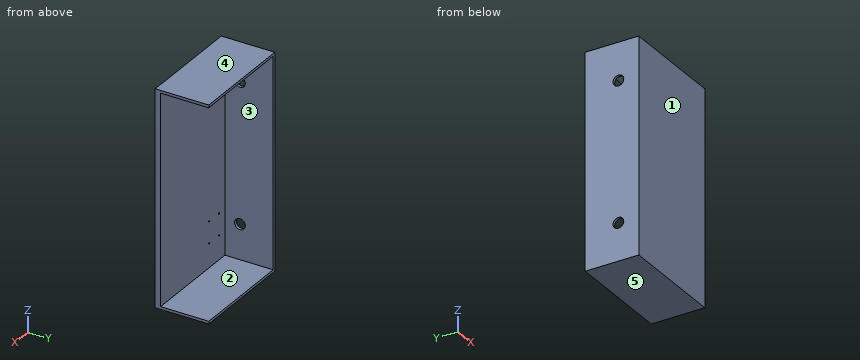
```python
from build123d import *

# Parameters (mm, degrees)
ESQUISSE1_W             = 200
ESQUISSE1_H             = 400
BOSS_EXTRU_1_DEPTH      = 10
BOSS_EXTRU_2_DEPTH      = 90
ENL_V_MAT_EXTRU_1_REACH = 458.098
ESQUISSE3_R             = 10
ESQUISSE4_R             = 1.5
ENL_V_MAT_EXTRU_2_DEPTH = 5


with BuildPart() as part:
    # Esquisse1 → Boss.-Extru.1 (new body)
    with BuildSketch(Plane(origin=(0, 0, 0), x_dir=(1, 0, 0), z_dir=(0, 1, 0))):
        with Locations((100, 200)):
            Rectangle(ESQUISSE1_W, ESQUISSE1_H)
    extrude(amount=BOSS_EXTRU_1_DEPTH)

    # Esquisse2 → Boss.-Extru.2 (add)
    with BuildSketch(Plane(origin=(0, 10, 0), x_dir=(1, 0, 0), z_dir=(0, 1, 0))):
        Polygon((5, 5), (5, 395), (200, 395), (200, 400), (0, 400), (0, 0), (200, 0), (200, 5), align=None)
    extrude(amount=BOSS_EXTRU_2_DEPTH)

    # Esquisse3 → Enlèv. mat.-Extru.1 (cut, up to next)
    with BuildSketch(Plane(origin=(5, 0, 0), x_dir=(0, 0, -1), z_dir=(1, 0, 0)), mode=Mode.PRIVATE) as enl_v_mat_extru_1_sk1:
        with Locations((70, 38)):
            Circle(ESQUISSE3_R)
    enl_v_mat_extru_1_tool1 = extrude(enl_v_mat_extru_1_sk1.sketch, amount=-ENL_V_MAT_EXTRU_1_REACH, mode=Mode.PRIVATE) & part.part
    # Esquisse3 → Enlèv. mat.-Extru.1 (cut, up to next)
    with BuildSketch(Plane(origin=(5, 0, 0), x_dir=(0, 0, -1), z_dir=(1, 0, 0)), mode=Mode.PRIVATE) as enl_v_mat_extru_1_sk2:
        with Locations((330, 38)):
            Circle(ESQUISSE3_R)
    enl_v_mat_extru_1_tool2 = extrude(enl_v_mat_extru_1_sk2.sketch, amount=-ENL_V_MAT_EXTRU_1_REACH, mode=Mode.PRIVATE) & part.part
    add(enl_v_mat_extru_1_tool1.solids().sort_by_distance((5, 38, -70))[0], mode=Mode.SUBTRACT)
    add(enl_v_mat_extru_1_tool2.solids().sort_by_distance((5, 38, -330))[0], mode=Mode.SUBTRACT)

    # Esquisse4 → Enlèv. mat.-Extru.2 (cut)
    with BuildSketch(Plane(origin=(0, 10, 0), x_dir=(1, 0, 0), z_dir=(0, 1, 0))):
        with Locations(Location((23, 350, 0), (0, 0, 270))):
            Circle(ESQUISSE4_R)
        with Locations(Location((53, 350, 0), (0, 0, 270))):
            Circle(ESQUISSE4_R)
        with Locations(Location((53, 310, 0), (0, 0, 270))):
            Circle(ESQUISSE4_R)
        with Locations(Location((23, 310, 0), (0, 0, 270))):
            Circle(ESQUISSE4_R)
        with Locations(Location((23, 90, 0), (0, 0, 90))):
            Circle(ESQUISSE4_R)
        with Locations(Location((53, 90, 0), (0, 0, 90))):
            Circle(ESQUISSE4_R)
        with Locations(Location((53, 50, 0), (0, 0, 90))):
            Circle(ESQUISSE4_R)
        with Locations(Location((23, 50, 0), (0, 0, 90))):
            Circle(ESQUISSE4_R)
    extrude(amount=-ENL_V_MAT_EXTRU_2_DEPTH, mode=Mode.SUBTRACT)


solid = part.part
```
Source: CAD feature listing. Evaluate the final solid. Frame: model axes, mm. Face numbers are marked on the shaded views. A direction names the side the tool comes from. Round coordinates to 2 decimals unless told otherwise and drop trailing zeros. Loops run counter-clockwise (first coordinate to the right, second up) from the corner with the lowest first, then second, coordinate; pieces in that order, holes last.
1. Section query C-C on x = 110.5. Output: boundary loops of the cut face in (y, z).
2. Section query B-B on z = -70. Output: boundary loops of the cut face in (x, y), and give its area (3 significant figures).
3. Mould query, pull axis Z, two halves, no side actions, for the marked faces 3, 4 and 5. Classes: released by +Z, released by -Z, zero draft, split by the parting line, or undercut.
4. Ray query, L1, parallel to X at y = 8.15, z = -350; L2, parallel to Z at x = 154, y = 26.5; L3, parallel to Y at x = 3, z = -330. Return the intervals inside material, ascending.
5. Contact query for flat-ended pins moving along their axis: pin 1 (10 mm diameter, centred on x = 150, z = -115, fed in from +Y); pin 2 (6 mm diameter, centred on y = 34.5, z = -62, fed in from -X); pin 3 (1.8 mm diameter, centred on x = 23, z = -90, fed in from +Y); pin 4 (8 mm diameter, centred on y = 79.5, z = -152.5, fed in from +X). Output: stop coordinate, or through.
6. Section query D-D on y = 76. Output: boundary loops of the cut face in (x, z).
7. Access query for the marked faces 1 and 2. Directions: +Z, -Z, +X, -X, +Y, -Y. A direction counts if a zero-diameter tool reaches every point of the face in a straight line with its end or side. Return the directions, or none.
8. Section query A-A on y = 38. Output: boundary loops of the cut face in (x, z), and give its area (3 significant figures).
Answers below:
1. outline: (0, -400) - (100, -400) - (100, -395) - (10, -395) - (10, -5) - (100, -5) - (100, 0) - (0, 0) - close
2. outline: (0, 0) - (200, 0) - (200, 10) - (5, 10) - (5, 28) - (0, 28) - close; (0, 48) - (5, 48) - (5, 100) - (0, 100) - close
2. area: 2,350 mm2
3. face 3: undercut
3. face 4: released by +Z
3. face 5: released by -Z
4. L1: x = 0 to 21.5, 24.5 to 51.5, 54.5 to 200
4. L2: z = -400 to -395, -5 to 0
4. L3: y = 0 to 28, 48 to 100
5. pin 1: stops at y = 10
5. pin 2: stops at x = 0
5. pin 3: stops at y = 5
5. pin 4: stops at x = 5
6. outline: (0, -400) - (200, -400) - (200, -395) - (5, -395) - (5, -5) - (200, -5) - (200, 0) - (0, 0) - close
7. face 1: +Z, -Z, +X, -X, -Y
7. face 2: +X, +Y
8. outline: (0, -400) - (200, -400) - (200, -395) - (5, -395) - (5, -340) - (0, -340) - close; (0, -320) - (5, -320) - (5, -80) - (0, -80) - close; (0, -60) - (5, -60) - (5, -5) - (200, -5) - (200, 0) - (0, 0) - close
8. area: 3,750 mm2
